from build123d import *

# Parameters (mm, degrees)
SKETCH1_R           = 44
BOSS_EXTRUDE1_DEPTH = 160
BOSS_EXTRUDE2_DEPTH = 12
SKETCH5_R           = 6.5
CUT_EXTRUDE3_DEPTH  = 80
SKETCH6_R           = 35
CUT_EXTRUDE4_DEPTH  = 142
SKETCH7_R           = 25.5
CUT_EXTRUDE5_DEPTH  = 82


with BuildPart() as part:
    # Sketch1 → Boss-Extrude1 (new body)
    with BuildSketch(Plane(origin=(0, 0, 0), x_dir=(0, 0, -1), z_dir=(1, 0, 0))):
        Circle(SKETCH1_R)
    extrude(amount=BOSS_EXTRUDE1_DEPTH)

    # Sketch2 → Boss-Extrude2 (add)
    with BuildSketch(Plane(origin=(160, 0, 0), x_dir=(0, 0, -1), z_dir=(1, 0, 0))):
        with BuildLine():
            Line((-25.925925926, 42.753319928), (-75.277777778, 12.825995978))
            ThreePointArc((-75.277777778, 12.825995978), (-82.5, 0), (-75.277777778, -12.825995978))
            Line((-75.277777778, -12.825995978), (-25.925925926, -42.753319928))
            ThreePointArc((-25.925925926, -42.753319928), (0, -50), (25.925925926, -42.753319928))
            Line((25.925925926, -42.753319928), (75.277777778, -12.825995978))
            ThreePointArc((75.277777778, -12.825995978), (82.5, 0), (75.277777778, 12.825995978))
            Line((75.277777778, 12.825995978), (25.925925926, 42.753319928))
            ThreePointArc((25.925925926, 42.753319928), (0, 50), (-25.925925926, 42.753319928))
        make_face()
    extrude(amount=BOSS_EXTRUDE2_DEPTH)

    # Sketch5 → Cut-Extrude3 (cut)
    with BuildSketch(Plane(origin=(172, 0, 0), x_dir=(0, 0, -1), z_dir=(1, 0, 0))):
        with Locations((67.5, 0)):
            Circle(SKETCH5_R)
        with Locations((-67.5, 0)):
            Circle(SKETCH5_R)
    extrude(amount=-CUT_EXTRUDE3_DEPTH, mode=Mode.SUBTRACT)

    # Sketch6 → Cut-Extrude4 (cut)
    with BuildSketch(Plane(origin=(172, 0, 0), x_dir=(0, 0, -1), z_dir=(1, 0, 0))):
        Circle(SKETCH6_R)
    extrude(amount=-CUT_EXTRUDE4_DEPTH, mode=Mode.SUBTRACT)

    # Sketch7 → Cut-Extrude5 (cut)
    with BuildSketch(Plane.ZY):
        Circle(SKETCH7_R)
    extrude(amount=-CUT_EXTRUDE5_DEPTH, mode=Mode.SUBTRACT)

    # Sketch9 → Cut-Revolve1 (revolve, cut)
    with BuildSketch(Plane(origin=(0, 0, 0), x_dir=(1, 0, 0), z_dir=(0, 1, 0)), mode=Mode.PRIVATE) as cut_revolve1_sk:
        Polygon((30, 38.002095215), (23.999999428, 44.002095215), (35.999999428, 44.002095215), align=None)
        Polygon((160, 44.000612252), (160, 38.000612252), (154, 44.000612252), align=None)
    revolve(cut_revolve1_sk.sketch.rotate(Axis((0, 0, 0), (1, 0, 0)), 180), axis=Axis((0, 0, 0), (1, 0, 0)), mode=Mode.SUBTRACT)


solid = part.part
Can you work these out from the model? Positions are in its coordinate system, mm. A direction names the side the tool comes from. Give positions to 0.01 mm unless a question says otherwise; leave off trailing zeros. Loops run counter-clockwise (first coordinate to the right, second up) from the corner with the lowest first, then second, coordinate; pieces in that order, holes last. Notation, with made-up numbers: (63, 1) -> (79, 1) arc R26 ccw to (79, 15) -> close; hole circle Ø3 at (6, 14). An arc over 180 degrees is marked (long way). Use one line per item in the form item = value.
1) We'd pull the mould along Y, two halves only. Please class faces 5 (the face through (30, -26, -2)), 6 (the face through (165.916, 27.999, 50.256)), 7 (the face through (166.08, 1.95, 61.3)), 8 (the face through (172, 1, 38)): released by +Y, released by -Y, zero draft, split by the parting line, or undercut.
Answers:
face_5 = undercut
face_6 = released by +Y
face_7 = undercut
face_8 = zero draft
2) If we section it at B-B (x = 81.5): Please give me the cut outline in (y, z).
Answers:
outline = circle Ø88 at (0, 0); hole circle Ø70 at (0, 0)
3) I need wall thicknesses on line 1 along Z through (x, y) = (125.5, -1.5); line 2 along Y through (x, z) = (166, -67); line 3 along X through (y, z) = (-28, 19). Which ranges of each line are inside material? Lowest first, please.
Answers:
line_1 = -43.97 to -34.97, 34.97 to 43.97
line_2 = -17.85 to -6.48, 6.48 to 17.85
line_3 = 0 to 30
4) Will these pins go through, and if not, where does the flat tip stop? pin 1 (4 mm diameter, centred on x = 135.5, z = 35, fed in from -Y); pin 2 (21 mm diameter, centred on y = 14.5, z = -10, fed in from +X); pin 3 (8 mm diameter, centred on x = 118, y = 2.5, fed in from +Z).
Answers:
pin_1 = -29.1
pin_2 = 30
pin_3 = 44
5) If we section it at C-C (y = 0): Count the separate pieces of the cut face and the enclosed holes in it, plus the area to 3 significant figures.
Answers:
separate_pieces = 4
enclosed_holes = 0
area = 4,170 mm²
6) If we section it at A-A (z = 67.5): Please give me the cut outline in (x, y).
Answers:
outline = (160, -17.54) -> (172, -17.54) -> (172, -6.5) -> (160, -6.5) -> close; (160, 6.5) -> (172, 6.5) -> (172, 17.54) -> (160, 17.54) -> close
7) For faces 1 (the face through (166, 50, 0)), 2 (the face through (102, -21, 28)), 3 (the face through (159.625, 37.463, -8.319)), 4 (the face through (11.833, -42.954, 9.538)), which set-ups out of +Z, -Z, +X, -X, +Y, -Y let a thin tool reach every point of the face, with its end or its side?
Answers:
face_1 = +X, -X, +Y
face_2 = +X
face_3 = none
face_4 = -X
8) If we section it at D-D (z = -67): Please give me the cut outline in (x, y).
Answers:
outline = (160, -17.85) -> (172, -17.85) -> (172, -6.48) -> (160, -6.48) -> close; (160, 6.48) -> (172, 6.48) -> (172, 17.85) -> (160, 17.85) -> close
